```python
from build123d import *

# Parameters (mm, degrees)
SKETCH2_W           = 94.275056846
SKETCH2_H           = 59.98986983
SKETCH2_W_2         = 89.195056846
SKETCH2_H_2         = 54.90986983
REVOLVE_THIN1_ANGLE = 200


with BuildPart() as part:
    # Sketch2 → Revolve-Thin1 (revolve)
    with BuildSketch(Plane.XY):
        with Locations((-34.686966551, 11.785533037)):
            Rectangle(SKETCH2_W, SKETCH2_H)
        with Locations((-34.686966551, 11.785533037)):
            Rectangle(SKETCH2_W_2, SKETCH2_H_2, mode=Mode.SUBTRACT)
    revolve(axis=Axis((42.052924699, 43.793969352, 0), (0, -1, 0)), revolution_arc=REVOLVE_THIN1_ANGLE)


solid = part.part
```
Check sheet for the modelled part. Datum: model origin and axes. Units: mm. A direction names the side the tool comes from. Give positions to 0.01 mm unless a question says otherwise; leave off trailing zeros. Order: outer loops, then holes, each group sorted by start corner. A loop starts at its lowest first (then second) coordinate and runs counter-clockwise, first axis right, second up. Notation, with made-up numbers: M -38.75,-26.5 L -12.75,-26.5 A38 cw -12.75,12.5 Z; hole C 86,40.5 d4. An arc over 180 degrees is marked long. Answer in a Markdown table with one row per item. Add a question column.
Q1. Thickness scan on L1, parallel to Y at x = 123.5, z = -49.5; L2, parallel to Z at x = 67, y = 13.5; L3, parallel to X at y = 10, z = -103.5. Record the ranges inside material, lowest first.
Q2. Access from +Z, -Z, +X, -X, +Y, -Y to the whole of each face (thin tool, end or side, straight path). Record for faces 1 (the flat face through (-38, -17, 0)), 2 (the flat face through (44, 39.24, -41)), 3 (the flat face through (44, 41.78, -42)).
Q3. Sectioned sample at D-D, the plane z = -45. Record the boundary of the cut face in (x, y), and give its area (3 significant figures).
Q4. Gauge pin test, flat ends, axial feed: pin 1 Ø5 at (x, y) = (30, 28.5) entering from -Z; pin 2 Ø3 at (x, y) = (-50, 0.5) entering from +Z; pin 3 Ø1 at (x, y) = (60.5, 9.5) entering from -Z. Record the tip position at first contact, or that the pin passes through.
Q5. Sectioned sample at B-B, the plane z = -23. Record the boundary of the cut face in (x, y).
Q6. Sectioned sample at C-C, the plane x = 52. Record the boundary of the cut face in (y, z), and give its area (3 significant figures).
Q7. Sectioned sample at A-A, the plane y = 1.5. Record the boundary of the cut face in (x, z), and give its area (3 significant figures).
Q8. Release check for a two-part mould opening along X. For faces 4 (the cylindrical face through (46.86, 12.17, -31.78)), 5 (the cylindrical face through (60.577, 12.205, -122.485)), 6 (the flat face through (44, -18.209, -42)), 7 (the cylindrical face through (60.197, 12.17, -119.973)) record: released by +X, released by -X, zero draft, split by the parting line, or undercut.
Verdict:
| question | item | result |
|---|---|---|
| 1 | L1 | -18.21 to -15.67, 39.24 to 41.78 |
| 1 | L2 | -121.34 to -118.75, -20.27 to -15.94 |
| 1 | L3 | -26.02 to -21.28, 105.38 to 110.12 |
| 2 | face 1 | +Z, -X, +Y, -Y |
| 2 | face 2 | none |
| 2 | face 3 | +Z, -Z, +X, -X, +Y |
| 3 | outline | M -73.36,-18.21 L 157.47,-18.21 L 157.47,41.78 L -73.36,41.78 Z; hole M -70.63,-15.67 L 154.74,-15.67 L 154.74,39.24 L -70.63,39.24 Z |
| 3 | area | 1,470 mm² |
| 4 | pin 1 | z = -123.51 |
| 4 | pin 2 | z = -77.27 |
| 4 | pin 3 | z = -122.57 |
| 5 | outline | M -79.67,-18.21 L 23.42,-18.21 L 23.42,41.78 L -79.67,41.78 Z; M 60.69,-18.21 L 163.78,-18.21 L 163.78,41.78 L 60.69,41.78 Z; hole M -77.08,-15.67 L 19.6,-15.67 L 19.6,39.24 L -77.08,39.24 Z; hole M 64.51,-15.67 L 161.19,-15.67 L 161.19,39.24 L 64.51,39.24 Z |
| 6 | outline | M -18.21,-123.48 L 41.78,-123.48 L 41.78,-27.88 L -18.21,-27.88 Z; hole M -15.67,-120.93 L 39.24,-120.93 L 39.24,-30.56 L -15.67,-30.56 Z |
| 6 | area | 773 mm² |
| 7 | outline | M -81.82,0 A123.88 ccw long 158.46,42.37 L 156.07,41.5 A121.34 cw long -79.28,0 Z; M 9.91,0 A32.14 ccw long 72.26,10.99 L 69.87,10.12 A29.6 cw long 12.45,0 Z |
| 7 | area | 1,360 mm² |
| 8 | face 4 | undercut |
| 8 | face 5 | split by the parting line |
| 8 | face 6 | zero draft |
| 8 | face 7 | undercut |
